Here's how the part is built. I have some questions about the finished solid (model axes, mm). Give positions to 0.01 mm unless a question says otherwise; leave off trailing zeros. Write each loop counter-clockwise with the first axis right and the second up, starting at its lowest first coordinate (ties: lowest second). Pieces come first, ordered by that corner, then holes. Notation, with made-up numbers: (-34, 63.5) -> (-14, 63.5) arc R15 ccw to (-14, 84.5) -> close; hole circle Ø11 at (-8, 22.5). An arc over 180 degrees is marked (long way). Return JSON: item names as keys, results as strings.
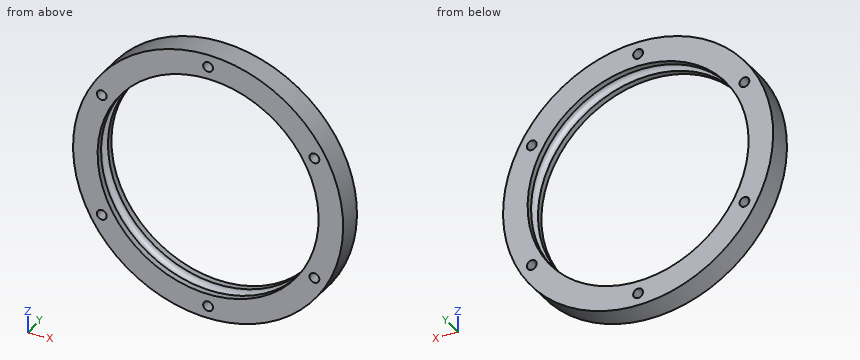
from build123d import *

# Parameters (mm, degrees)
CROQUIS2_R            = 2
CORTAR_EXTRUIR1_DEPTH = 10


with BuildPart() as part:
    # Croquis1 → Revolución1 (revolve)
    with BuildSketch(Plane(origin=(0, 0, 0), x_dir=(0, 0, -1), z_dir=(1, 0, 0))):
        with BuildLine():
            Line((-45, 2.5), (-45, 5))
            Line((-45, 5), (-55, 5))
            Line((-55, 5), (-55, -5))
            Line((-55, -5), (-45, -5))
            Line((-45, -5), (-45, -2.5))
            ThreePointArc((-45, -2.5), (-47.5, 0), (-45, 2.5))
        make_face()
    revolve(axis=Axis((0, 59.07084426, 0), (0, -1, 0)))

    # Croquis2 → Cortar-Extruir1 (cut)
    with BuildSketch(Plane(origin=(0, 5, 0), x_dir=(1, 0, 0), z_dir=(0, 1, 0))):
        with Locations(Location((0, 50, 0), (0, 0, 270))):
            Circle(CROQUIS2_R)
        with Locations(Location((43.301270189, 25, 0), (0, 0, 270))):
            Circle(CROQUIS2_R)
        with Locations(Location((43.301270189, -25, 0), (0, 0, 270))):
            Circle(CROQUIS2_R)
        with Locations(Location((0, -50, 0), (0, 0, 270))):
            Circle(CROQUIS2_R)
        with Locations(Location((-43.301270189, -25, 0), (0, 0, 270))):
            Circle(CROQUIS2_R)
        with Locations(Location((-43.301270189, 25, 0), (0, 0, 270))):
            Circle(CROQUIS2_R)
    extrude(amount=-CORTAR_EXTRUIR1_DEPTH, mode=Mode.SUBTRACT)


solid = part.part
1. Suppose I cut it at D-D, the plane z = 25. Count the separate pieces of the cut face and the enclosed holes in it, and give its area (3 significant figures).
Taken from the geometry:
{"separate pieces": "4", "enclosed holes": "0", "area": "128 mm²"}
2. For pin 1 Ø6.5 at (x, z) = (43.3, -25) entering from +Y; pin 2 Ø5 at (y, z) = (3.5, 20.5) entering from +X; pin 3 Ø3 at (x, y) = (13.5, -1.5) entering from +Z; pin 4 Ø2 at (x, y) = (-31.5, 2.5) entering from +Z, each with a flat end and sliding along its axis, tell me the tip position at first contact or that it passes through.
Taken from the geometry:
{"pin 1": "stops at y = 5", "pin 2": "stops at x = 51.97", "pin 3": "stops at z = 53.67", "pin 4": "stops at z = 45.77"}
3. Suppose I cut it at B-B, the plane z = 0. List the corners of the cut face in (x, y) for me.
Taken from the geometry:
{"outline": "(-55, -5) -> (-45, -5) -> (-45, -2.5) arc R2.5 cw to (-45, 2.5) -> (-45, 5) -> (-55, 5) -> close; (45, -5) -> (55, -5) -> (55, 5) -> (45, 5) -> (45, 2.5) arc R2.5 cw to (45, -2.5) -> close"}
4. Suppose I cut it at C-C, the plane y = 1.25. List the corners of the cut face in (x, z) for me.
Taken from the geometry:
{"outline": "circle Ø110 at (0, 0); hole circle Ø94.33 at (0, 0); hole circle Ø4 at (-43.3, -25); hole circle Ø4 at (-43.3, 25); hole circle Ø4 at (0, -50); hole circle Ø4 at (0, 50); hole circle Ø4 at (43.3, -25); hole circle Ø4 at (43.3, 25)"}
5. Suppose I cut it at A-A, the plane x = 0. List the corners of the cut face in (y, z) for me, and give its area (3 significant figures).
Taken from the geometry:
{"outline": "(-5, -55) -> (5, -55) -> (5, -52) -> (-5, -52) -> close; (-5, -48) -> (5, -48) -> (5, -45) -> (2.5, -45) arc R2.5 cw to (-2.5, -45) -> (-5, -45) -> close; (-5, 45) -> (-2.5, 45) arc R2.5 cw to (2.5, 45) -> (5, 45) -> (5, 48) -> (-5, 48) -> close; (-5, 52) -> (5, 52) -> (5, 55) -> (-5, 55) -> close", "area": "100 mm²"}
6. If I drill on line 1 (X direction, y = 2.75, z = -50); line 2 (X direction, y = -3.25, z = 16.5); line 3 (Z direction, x = -15, y = -1.5), over which ranges is the centre line in solid material (lowest first)? Write a range as [from, to].
Taken from the geometry:
{"line 1": "x = [-22.91, -2], [2, 22.91]", "line 2": "x = [-52.47, -41.87], [41.87, 52.47]", "line 3": "z = [-52.92, -44.54], [44.54, 52.92]"}
